Read the model definition and answer for the solid it produces. Units are mm, in the model's axes. A direction names the side the tool comes from. Round coordinates to 2 decimals unless told otherwise and drop trailing zeros. Order: outer loops, then holes, each group sorted by start corner. A loop starts at its lowest first (then second) coordinate and runs counter-clockwise, first axis right, second up. Notation, with made-up numbers: (15, 79) - (65, 79) arc R17 cw to (65, 97) - close; hole circle Ø10 at (70.5, 5). An arc over 180 degrees is marked (long way). Put each result on its own line as item: value. Start each with the question number.
Q1. Section C-C on x = 31.5 is taken. Give the vertices of the cut face in (y, z) (3 decimals).
Q2. Section A-A on z = 39.5 is taken. Give the vertices of the cut face in (x, y) (3 decimals).
Q3. Section B-B on y = -1 is taken. Give the vertices of the cut face in (x, z) (3 decimals), then the cut area to 3 significant figures.
Q4. This flat-tipped pin is pushed along its axis until it touches: pin 1 Ø1.5 at (x, y) = (0, -4) entering from +Z (3 decimals). Where does it stop, or does it pass through?
Q5. For a pull along X with two mould halves and no side action, classify faces 1 (the face through (-1, 0, 3.175)), 2 (the face through (49.272, 36.651, 25.756)), 3 (the face through (-50.8, 0, 25)) as pulls with the +X half, pulls with the -X half, needs draft (parallel to the pull), parting line crosses it, or undercut.
Q6. Which of the six approach directions +Z, -Z, +X, -X, +Y, -Y give full straight-line access (tool end or side, diameter ignored) to faces 4 (the face through (-1, -38.1, 25)), 5 (the face through (-47.625, 0, 27))?
Q7. Find the intervals of material crossed by line 1 along X through (y, z) = (-19.5, 7.5) (3 decimals); line 2 along Y through (x, z) = (-15.5, 43.5) (3 decimals); line 3 along Z through (x, y) = (-39.5, 2.5) (3 decimals), in increasing order. Write a range as from..to.
from build123d import *

# Parameters (mm, degrees)
F0_W     = 101.6
F0_H     = 76.2
F0_W_2   = 95.25
F0_H_2   = 69.85
F1_DEPTH = 50.8
F2_DEPTH = 3.175
F3_R     = 5.08


with BuildPart() as f1:
    # F0 (on Top) → F1 (new body)
    with BuildSketch(Plane.XY):
        Rectangle(F0_W, F0_H)
        Rectangle(F0_W_2, F0_H_2, mode=Mode.SUBTRACT)
    extrude(amount=F1_DEPTH)

    # F0 (on Top) → F2 (join)
    with BuildSketch(Plane.XY):
        Rectangle(F0_W_2, F0_H_2)
    extrude(amount=F2_DEPTH)

    # F3
    f3_edges = [f1.edges().sort_by_distance(p)[0] for p in [
        (50.8, 38.1, 25.4),
        (50.8, -38.1, 25.4),
        (-50.8, 38.1, 25.4),
        (-50.8, -38.1, 25.4),
    ]]
    fillet(f3_edges, radius=F3_R)


solid = f1.part
Findings:
1. outline: (-38.1, 0) - (38.1, 0) - (38.1, 50.8) - (34.925, 50.8) - (34.925, 3.175) - (-34.925, 3.175) - (-34.925, 50.8) - (-38.1, 50.8) - close
2. outline: (-50.8, -33.02) arc R5.08 ccw to (-45.72, -38.1) - (45.72, -38.1) arc R5.08 ccw to (50.8, -33.02) - (50.8, 33.02) arc R5.08 ccw to (45.72, 38.1) - (-45.72, 38.1) arc R5.08 ccw to (-50.8, 33.02) - close; hole (-47.625, -34.925) - (47.625, -34.925) - (47.625, 34.925) - (-47.625, 34.925) - close
3. outline: (-50.8, 0) - (50.8, 0) - (50.8, 50.8) - (47.625, 50.8) - (47.625, 3.175) - (-47.625, 3.175) - (-47.625, 50.8) - (-50.8, 50.8) - close
3. area: 625 mm2
4. pin 1: z = 3.175
5. face 1: undercut
5. face 2: pulls with the +X half
5. face 3: pulls with the -X half
6. face 4: +Z, -Z, +X, -X, -Y
6. face 5: +Z
7. line 1: -50.8..-47.625, 47.625..50.8
7. line 2: -38.1..-34.925, 34.925..38.1
7. line 3: 0..3.175
